For this review, use the dimensioned drawing (mm, ordinates from the lowest corner) and the shaded views. Coordinates: 2 decimals unless noted, no trailing zeros. Order: outer loops, then holes, each group sorted by start corner. A loop starts at its lowest first (then second) coordinate and runs counter-clockwise, first axis right, second up. Notation, with made-up numbers: M 57,67.25 L 103,67.25 A31 cw 103,98.25 Z; hole C -26,60.5 d4. An arc over 180 degrees is marked long. One line per item, written item: value.
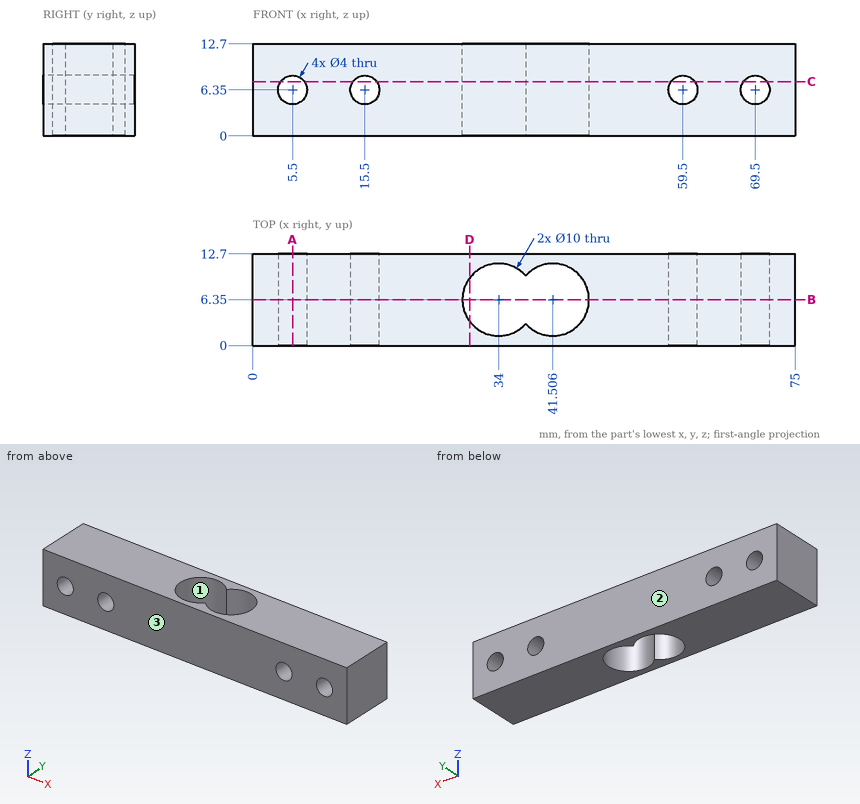
(1) Insertion check: pin 1 Ø3 at (x, z) = (69.5, 6.35) entering from +Y. The pin has a flat end and moves straight along its axis. Give the tip position at first contact, or say it passes through.
Geometry results:
pin 1: passes through
(2) For L1, parallel to X at y = 8.75, z = 6.35; L2, parallel to Y at x = 34, z = 8; L3, parallel to Z at x = 5.5, y = 5.75, list the stretches that pass through material, from the lowest coordinate up.
Geometry results:
L1: x = 0 to 3.5, 7.5 to 13.5, 17.5 to 29.61, 45.89 to 57.5, 61.5 to 67.5, 71.5 to 75
L2: y = 0 to 1.35, 11.35 to 12.7
L3: z = 0 to 4.35, 8.35 to 12.7
(3) Mouldability with a two-part tool opening along Y and no side actions: class the marked faces 1, 2 and 3 as +Y half, -Y half, draft (parallel to the pull), parting line (faces both ways), or undercut.
Geometry results:
face 1: undercut
face 2: +Y half
face 3: -Y half
(4) We need section D-D, the plane x = 30. State the section outline as (y, z) points, plus the area to 3 significant figures.
Geometry results:
outline: M 0,0 L 3.35,0 L 3.35,12.7 L 0,12.7 Z; M 9.35,0 L 12.7,0 L 12.7,12.7 L 9.35,12.7 Z
area: 85.1 mm2
(5) We need section A-A, the plane x = 5.5. State the section outline as (y, z) points, plus the area to 4 significant figures.
Geometry results:
outline: M 0,0 L 12.7,0 L 12.7,4.35 L 0,4.35 Z; M 0,8.35 L 12.7,8.35 L 12.7,12.7 L 0,12.7 Z
area: 110.5 mm2
(6) We need section B-B, the plane y = 6.35. State the section outline as (x, z) points, plus the area to 3 significant figures.
Geometry results:
outline: M 0,0 L 29,0 L 29,12.7 L 0,12.7 Z; M 46.51,0 L 75,0 L 75,12.7 L 46.51,12.7 Z; hole C 5.5,6.35 d4; hole C 15.5,6.35 d4; hole C 59.5,6.35 d4; hole C 69.5,6.35 d4
area: 680 mm2
(7) We need section C-C, the plane z = 7.5. State the section outline as (x, y) points.
Geometry results:
outline: M 0,0 L 3.86,0 L 3.86,12.7 L 0,12.7 Z; M 7.14,0 L 13.86,0 L 13.86,12.7 L 7.14,12.7 Z; M 17.14,0 L 57.86,0 L 57.86,12.7 L 17.14,12.7 Z; M 61.14,0 L 67.86,0 L 67.86,12.7 L 61.14,12.7 Z; M 71.14,0 L 75,0 L 75,12.7 L 71.14,12.7 Z; hole M 37.75,3.05 A5 ccw long 37.75,9.65 A5 ccw long Z
